Read the model definition and answer for the solid it produces. Units are mm, in the model's axes. Coordinates: 2 decimals unless noted, no trailing zeros. Loops run counter-clockwise (first coordinate to the right, second up) from the corner with the lowest first, then second, coordinate; pieces in that order, holes last.
Autodesk Inventor part; units mm, degrees
ref_plane "YZ Plane" through (0, 0, 0) normal (1, 0, 0) x (0, 1, 0)
ref_plane "XZ Plane" through (0, 0, 0) normal (0, 1, 0) x (-1, 0, 0)
ref_plane "XY Plane" through (0, 0, 0) normal (0, 0, 1) x (1, 0, 0)
sketch "Sketch1" plane through (0, 0, 0) normal (0, 1, 0) x (-1, 0, 0)
  line L0 (0, 0) -> (130, 0)
  line L1 (130, 0) -> (130, -120)
  line L2 (130, -120) -> (0, -120)
  line L3 (0, -120) -> (0, 0)
  dimension "d0" = 120
  dimension "d1" = 130
extrude "Extrusion1" add sketch "Sketch1" along normal blind 10
sketch "Sketch2" plane through (0, 10, 0) normal (0, 1, 0) x (1, 0, 0)
  circle A0 centre (-120, 110) radius 4.7625
  line L0 (-130, 120) -> (-130, 0)
  line L1 (0, 120) -> (-130, 120)
  point P0 (0, 0)
  dimension "d4" = 10
  dimension "d5" = 10
  dimension "d6" = 9.525
extrude "Extrusion2" cut sketch "Sketch2" against normal blind 10
ref_plane "Work Plane1" through (-65, 0, 0) normal (1, 0, 0) x (0, 0, -1)
ref_plane "Work Plane2" through (0, 0, -60) normal (0, 0, -1) x (-1, 0, 0)
mirror "Mirror1" about plane through (0, 0, -60) normal (0, 0, -1) of "Extrusion2"
mirror "Mirror2" about plane through (-65, 0, 0) normal (1, 0, 0) of "Extrusion2", "Mirror1"
properties part number "Bottom_part"
Item 1: Find the intervals of material crossed by line 1 along Z through (x, y) = (-120, 2.75); line 2 along X through (y, z) = (5.25, -110); line 3 along Z through (x, y) = (-118, 2.5), in increasing order.
Numbers:
line 1: z = -120 to -114.76, -105.24 to -14.76, -5.24 to 0
line 2: x = -130 to -124.76, -115.24 to -14.76, -5.24 to 0
line 3: z = -120 to -114.32, -105.68 to -14.32, -5.68 to 0
Item 2: A cutting plane is placed at A-A on z = -110. Determine the outline of the cut face in (x, y).
Numbers:
outline: (-130, 0) - (-124.76, 0) - (-124.76, 10) - (-130, 10) - close; (-115.24, 0) - (-14.76, 0) - (-14.76, 10) - (-115.24, 10) - close; (-5.24, 0) - (0, 0) - (0, 10) - (-5.24, 10) - close
Item 3: Determine the mould class of faces 1 (the face through (-130, 5, -59)), 2 (the face through (-64, 5, 0)), 3 (the face through (-9.38, 5.07, -105.28)) for opening direction X: released by +X, released by -X, zero draft, split by the parting line, or undercut.
Numbers:
face 1: released by -X
face 2: zero draft
face 3: undercut
Item 4: A cutting plane is placed at C-C on x = -10. Determine the outline of the cut face in (y, z).
Numbers:
outline: (0, -120) - (10, -120) - (10, -114.76) - (0, -114.76) - close; (0, -105.24) - (10, -105.24) - (10, -14.76) - (0, -14.76) - close; (0, -5.24) - (10, -5.24) - (10, 0) - (0, 0) - close
Item 5: A cutting plane is placed at B-B on y = 7.5. Determine the outline of the cut face in (x, z) (1 decimal).
Numbers:
outline: (-130, -120) - (0, -120) - (0, 0) - (-130, 0) - close; hole circle Ø9.5 at (-120, -110); hole circle Ø9.5 at (-120, -10); hole circle Ø9.5 at (-10, -110); hole circle Ø9.5 at (-10, -10)
